```python
from build123d import *

# Parameters (mm, degrees)
SKETCH_1_R          = 2.5
EXTRUDE_1_DEPTH     = 88
CUT_EXTRUDE_1_DEPTH = 22


with BuildPart() as part:
    # 스케치1 → 보스-돌출1 (new body)
    with BuildSketch(Plane.XY):
        Circle(SKETCH_1_R)
    extrude(amount=EXTRUDE_1_DEPTH)

    # 스케치2 → 컷-돌출1 (cut)
    with BuildSketch(Plane(origin=(0, 0, 0), x_dir=(-1, 0, 0), z_dir=(0, 0, -1))):
        with BuildLine():
            Line((1.5, 2), (-1.5, 2))
            ThreePointArc((-1.5, 2), (0, 2.5), (1.5, 2))
        make_face()
    cut_extrude_1 = extrude(amount=-CUT_EXTRUDE_1_DEPTH, mode=Mode.SUBTRACT)

    # 대칭 복사1: 컷-돌출1 across plane
    add(cut_extrude_1.mirror(Plane(origin=(0, 0, 44), x_dir=(1, 0, 0), z_dir=(0, 0, -1))), mode=Mode.SUBTRACT)


solid = part.part
```
Can you work these out from the model? Positions are in its coordinate system, mm. A direction names the side the tool comes from. Coordinates: 2 decimals unless noted, no trailing zeros. Loops run counter-clockwise (first coordinate to the right, second up) from the corner with the lowest first, then second, coordinate; pieces in that order, holes last. Notation, with made-up numbers: (63, -23) -> (91, -23) arc R8 cw to (91, -19) -> close; hole circle Ø2 at (55, 38). An arc over 180 degrees is marked (long way). Put each result on its own line as item: value. Start each with the question number.
Q1. I want a section at B-B (z = 71). Write out the boundary of the cut face in (x, y).
Q2. I'm going to push flat-ended pins straight in: P1, Ø1, axis at x = 1.5, z = 59, coming from the +Y side; P2, Ø1, axis at x = -1, z = 23.5, coming from the -Y side. Where does each tip first touch, or does it pass through?
Q3. For faces 1 (the face through (0, 0, 88)), 2 (the face through (0, 2, 77)), 3 (the face through (0, 2, 11)), which set-ups out of +Z, -Z, +X, -X, +Y, -Y let a thin tool reach every point of the face, with its end or its side?
Q4. I want a section at C-C (y = 1). Write out the boundary of the cut face in (x, z).
Q5. If I drill on line 1 (Z direction, x = -0.6, y = 2.3); line 2 (X direction, y = -0.2, z = 60), over which ranges is the centre line in solid material (lowest first)? Write a range as [from, to].
Q6. I want a section at A-A (x = 0). Write out the boundary of the cut face in (y, z).
Taken from the geometry:
1. outline: (-1.5, 2) arc R2.5 ccw (long way) to (1.5, 2) -> close
2. P1: stops at y = 2.29
2. P2: stops at y = -2.45
3. face 1: +Z, +X, -X, +Y, -Y
3. face 2: +Z, +X, -X, +Y
3. face 3: -Z, +X, -X, +Y
4. outline: (-2.29, 0) -> (2.29, 0) -> (2.29, 88) -> (-2.29, 88) -> close
5. line 1: z = [22, 66]
5. line 2: x = [-2.49, 2.49]
6. outline: (-2.5, 0) -> (2, 0) -> (2, 22) -> (2.5, 22) -> (2.5, 66) -> (2, 66) -> (2, 88) -> (-2.5, 88) -> close
